```python
from build123d import *

# Parameters (mm, degrees)
BOSS_EXTRUDE1_START = 15.549813
SKETCH1_W           = 90
SKETCH1_H           = 100
SKETCH1_R           = 2.5
SKETCH1_R_2         = 3.57
BOSS_EXTRUDE1_DEPTH = 3.18
BOSS_EXTRUDE2_DEPTH = 3.18
SKETCH3_R           = 1.5
SKETCH3_R_2         = 15.5
CUT_EXTRUDE1_DEPTH  = 10
FILLET1_R           = 10


with BuildPart() as part:
    # Sketch1 → Boss-Extrude1 (new body)
    with BuildSketch(Plane.XY.offset(BOSS_EXTRUDE1_START)):
        with Locations((0, -5)):
            Rectangle(SKETCH1_W, SKETCH1_H)
        with Locations((32.3, -42.3)):
            Circle(SKETCH1_R, mode=Mode.SUBTRACT)
        with Locations((-32.3, -42.3)):
            Circle(SKETCH1_R_2, mode=Mode.SUBTRACT)
        with Locations((-32.3, 32.3)):
            Circle(SKETCH1_R_2, mode=Mode.SUBTRACT)
        with Locations((32.3, 32.3)):
            Circle(SKETCH1_R, mode=Mode.SUBTRACT)
    extrude(amount=BOSS_EXTRUDE1_DEPTH)

    # Sketch2 → Boss-Extrude2 (add, through all)
    with BuildSketch(Plane.XY.offset(18.729812892)):
        Polygon((45, 45), (68.012220348, 16.59), (68.012220348, -26.59), (45, -55), align=None)
    extrude(amount=-BOSS_EXTRUDE2_DEPTH)

    # Sketch3 → Cut-Extrude1 (cut)
    with BuildSketch(Plane.XY.offset(18.729812892)):
        with Locations((29.5, 10.5)):
            Circle(SKETCH3_R)
        with Locations((60.5, 10.5)):
            Circle(SKETCH3_R)
        with Locations((60.5, -20.5)):
            Circle(SKETCH3_R)
        with Locations((29.5, -20.5)):
            Circle(SKETCH3_R)
        with Locations((45, -5)):
            Circle(SKETCH3_R_2)
    extrude(amount=-CUT_EXTRUDE1_DEPTH, mode=Mode.SUBTRACT)

    # Fillet1
    fillet1_edges = [part.edges().sort_by_distance(p)[0] for p in [
        (68.012220348, 16.59, 17.139812892),
        (68.012220348, -26.59, 17.139812892),
        (-45, 45, 17.139813),
        (45, 45, 17.139813),
        (45, -55, 17.139813),
        (-45, -55, 17.139813),
    ]]
    fillet(fillet1_edges, radius=FILLET1_R)


solid = part.part
```
Geometry check sheet. Reference: the model listing, model coordinates, mm. Coordinates: 2 decimals unless noted, no trailing zeros. Write each loop counter-clockwise with the first axis right and the second up, starting at its lowest first coordinate (ties: lowest second). Pieces come first, ordered by that corner, then holes. Notation, with made-up numbers: M 77,-12.5 L 129,-12.5 A26 cw 129,12.5 Z; hole C 40.25,-5.5 d1. An arc over 180 degrees is marked long. Use one line per item in the form item = value. Start each with the question number.
1) Go/stop test with flat-tipped pins: pin 1 Ø6.5 at (x, y) = (-32.3, -42.3) entering from -Z; pin 2 Ø4 at (x, y) = (29.5, -20.5) entering from +Z. Record where each tip stops, or that it passes through.
2) Release check for a two-part mould opening along Y. For faces 1 (the flat face through (57.02, -40.16, 17.16)), 2 (the cylindrical face through (34.61, 31.34, 17.12)), 3 (the flat face through (68.012, -5, 17)) record: pulls with the +Y half, pulls with the -Y half, needs draft (parallel to the pull), parting line crosses it, or undercut.
3) Thickness scan on probe 1 along Y at (x, z) = (-32.3, 17.4); probe 2 along Y at (x, z) = (32.5, 17.1); probe 3 along Y at (x, z) = (32.3, 17.45). Record the ranges inside material, lowest first. Write a range as from..to.
4) Section check A-A on y = -5. Enter the section's corners in (x, z), and give its area (3 significant figures).
5) Section check D-D on y = -42.3. Enter the section's corners in (x, z).
6) Section check B-B on x = -32.3. Enter the section's corners in (y, z).
7) Section check C-C on z = 16.9. State how many separate pieces and enclosed holes the cut face has, and give its area (3 significant figures).
Responses:
q1.pin_1 = through
q1.pin_2 = 18.73
q2.face_1 = pulls with the -Y half
q2.face_2 = undercut
q2.face_3 = needs draft
q3.probe_1 = -55..-45.87, -38.73..28.73, 35.87..45
q3.probe_2 = -55..-44.79, -39.81..-14.17, 4.17..29.81, 34.79..45
q3.probe_3 = -55..-44.8, -39.8..-13.89, 3.89..29.8, 34.8..45
q4.outline = M -45,15.55 L 29.5,15.55 L 29.5,18.73 L -45,18.73 Z; M 60.5,15.55 L 68.01,15.55 L 68.01,18.73 L 60.5,18.73 Z
q4.area = 261 mm2
q5.outline = M -45,15.55 L -35.87,15.55 L -35.87,18.73 L -45,18.73 Z; M -28.73,15.55 L 29.8,15.55 L 29.8,18.73 L -28.73,18.73 Z; M 34.8,15.55 L 55.29,15.55 L 55.29,18.73 L 34.8,18.73 Z
q6.outline = M -55,15.55 L -45.87,15.55 L -45.87,18.73 L -55,18.73 Z; M -38.73,15.55 L 28.73,15.55 L 28.73,18.73 L -38.73,18.73 Z; M 35.87,15.55 L 45,15.55 L 45,18.73 L 35.87,18.73 Z
q7.separate_pieces = 1
q7.enclosed_holes = 9
q7.area = 9,690 mm2
